Could you check a few things on this drawing? It's one solid part, dimensions in mm from its lowest x, y, z. A direction names the side the tool comes from. Coordinates: 2 decimals unless noted, no trailing zeros. Write each loop counter-clockwise with the first axis right and the second up, starting at its lowest first coordinate (ties: lowest second). Pieces come first, ordered by that corner, then holes.
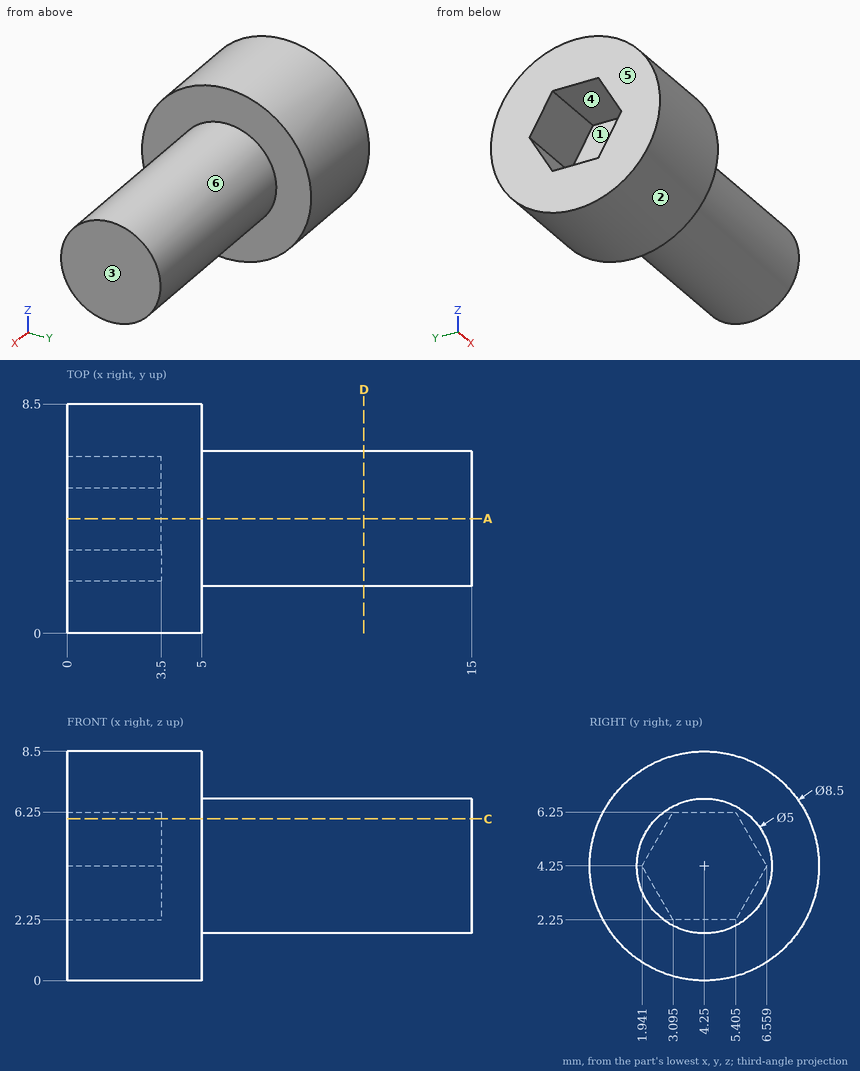
1) Imagine slicing it at C-C on z = 6. Please give me the cut outline in (x, y) (1 decimal).
Values follow:
outline: (0, 0.4) - (5, 0.4) - (5, 2.5) - (15, 2.5) - (15, 6) - (5, 6) - (5, 8.1) - (0, 8.1) - (0, 5.5) - (3.5, 5.5) - (3.5, 3) - (0, 3) - close
2) I need wall thicknesses on probe 1 along X at (y, z) = (2.75, 0.75); probe 2 along X at (y, z) = (5.75, 4.75); probe 3 along Y at (x, z) = (2.5, 2.5). Which ranges of each line are inside material? Lowest first, please.
Values follow:
probe 1: x = 0 to 5
probe 2: x = 3.5 to 15
probe 3: y = 0.38 to 2.95, 5.55 to 8.12
3) We'd pull the mould along Y, two halves only. Please class the marked faces 1, 2 and 3: pulls with the +Y half, pulls with the -Y half, needs draft (parallel to the pull), parting line crosses it, or undercut.
Values follow:
face 1: undercut
face 2: parting line crosses it
face 3: needs draft
4) Will these pins go through, and if not, where does the flat tip stop? pin 1 (3 mm diameter, centred on y = 4.5, z = 4, fed in from -X); pin 2 (1.5 mm diameter, centred on x = 7, z = 3.5, fed in from +Y); pin 3 (5 mm diameter, centred on x = 12.5, y = 4, fed in from +Z).
Values follow:
pin 1: stops at x = 3.5
pin 2: stops at y = 6.75
pin 3: stops at z = 6.75
5) Imagine slicing it at D-D on x = 11. Please give me the cut outline in (y, z), then the cut area to 3 significant figures.
Values follow:
outline: circle Ø5 at (4.25, 4.25)
area: 19.6 mm2
6) Imagine slicing it at A-A on y = 4.25. Please give me the cut outline in (x, z).
Values follow:
outline: (0, 0) - (5, 0) - (5, 1.75) - (15, 1.75) - (15, 6.75) - (5, 6.75) - (5, 8.5) - (0, 8.5) - (0, 6.25) - (3.5, 6.25) - (3.5, 2.25) - (0, 2.25) - close
7) On a 3-axis mill with a long thin cutter (end or side, diameter ignored), from which of +Z, -Z, +X, -X, +Y, -Y can I reach the whole of each face in a straight line? I mean the marked faces 4, 5 and 6. Say none if no direction works.
Values follow:
face 4: -X
face 5: +Z, -Z, -X, +Y, -Y
face 6: +X
